For this review, take the finished solid that the model builds, in its own axes (mm). A direction names the side the tool comes from. Coordinates: 2 decimals unless noted, no trailing zeros. Loops run counter-clockwise (first coordinate to the right, second up) from the corner with the lowest first, then second, coordinate; pieces in that order, holes last. Notation, with made-up numbers: (84.5, 59) -> (109.5, 59) arc R25 ccw to (109.5, 93) -> close; hole circle Ø1 at (-12.75, 21). An arc over 180 degrees is marked (long way). Answer in a Markdown table with one row per item.
from build123d import *

# Parameters (mm, degrees)
F0_W     = 50.8
F0_H     = 25.4
F1_DEPTH = 50.8


with BuildPart() as f1:
    # F0 (on Top) → F1 (new body)
    with BuildSketch(Plane.XY):
        with Locations((43.003823, 0.562944)):
            Rectangle(F0_W, F0_H)
        Polygon((-83.996177, 13.262944), (-83.996177, -62.937056), (-58.596177, -62.937056), (-58.596177, -12.137056), (17.603823, -12.137056), (17.603823, 13.262944), align=None)
    extrude(amount=F1_DEPTH)


solid = f1.part
Item 1: For L1, parallel to Y at x = 24, z = 15; L2, parallel to X at y = -52, z = 34.5, list the stretches that pass through material, from the lowest coordinate up.
Worked answers:
| item | result |
|---|---|
| L1 | -12.14 to 13.26 |
| L2 | -84 to -58.6 |
Item 2: Take a section at B-B, the plane y = -20.5. State the section outline as (x, z) points.
Worked answers:
| item | result |
|---|---|
| outline | (-84, 0) -> (-58.6, 0) -> (-58.6, 50.8) -> (-84, 50.8) -> close |
Item 3: For faces 1 (the flat face through (-58.596, -38, 25)), 2 (the flat face through (-83.996, -24, 25)), list the 3-axis set-ups (+Z, -Z, +X, -X, +Y, -Y) from which the entire face can be reached by the end or side of a thin tool; tool diameter is ignored.
Worked answers:
| item | result |
|---|---|
| face 1 | +Z, -Z, +X, -Y |
| face 2 | +Z, -Z, -X, +Y, -Y |
Item 4: Insertion check: pin 1 (10 mm diameter, centred on y = -19.5, z = 8, fed in from +X). The pin has a flat end and moves straight along its axis. Give the tip position at first contact, or say it passes through.
Worked answers:
| item | result |
|---|---|
| pin 1 | x = -58.6 |
Item 5: Take a section at A-A, the plane z = 26. State the section outline as (x, y) points.
Worked answers:
| item | result |
|---|---|
| outline | (-84, -62.94) -> (-58.6, -62.94) -> (-58.6, -12.14) -> (68.4, -12.14) -> (68.4, 13.26) -> (-84, 13.26) -> close |
Item 6: Take a section at C-C, the plane x = -2. State the section outline as (y, z) points, and give its area (3 significant figures).
Worked answers:
| item | result |
|---|---|
| outline | (-12.14, 0) -> (13.26, 0) -> (13.26, 50.8) -> (-12.14, 50.8) -> close |
| area | 1,290 mm² |
